The listing builds one solid part. Answer for the finished solid, in the listing's coordinates (mm). Face numbers are marked on the shaded views. A direction names the side the tool comes from. Give positions to 0.01 mm unless a question says otherwise; leave off trailing zeros. Write each loop counter-clockwise with the first axis right and the second up, starting at its lowest first coordinate (ties: lowest second). Pieces come first, ordered by that corner, then holes. Notation, with made-up numbers: (70, 85) -> (84, 85) arc R14 cw to (84, 111) -> close; hole circle Ø9 at (56, 27). An arc over 180 degrees is marked (long way). Put each result on its own line as item: value. Start each with the question number.
1) A cutting plane is placed at D-D (x = 5.25). Write down the section's boundary in (y, z) (3 decimals), then the cut area to 3 significant figures.
2) Find the intervals of material crossed by line 1 along Z through (x, y) = (0, -2); line 2 along Z through (x, y) = (0.5, -2.25); line 3 along Z through (x, y) = (5, 3.25), in increasing order. Write a range as from..to.
3) A cutting plane is placed at C-C (z = -3.5). Write down the section's boundary in (x, y).
4) Flat-ended cylindrical pins translate along their axes: pin 1 Ø6 at (x, z) = (0, -40.259) entering from -Y (3 decimals); pin 2 Ø1.5 at (x, y) = (2, -4) entering from -Z. Find the tip coordinate at first contact, or state that the pin passes through.
5) For a pull along Z with two mould halves and no side action, classify the marked faces 5, 6 and 7 as released by +Z, released by -Z, zero draft, split by the parting line, or undercut.
6) A cutting plane is placed at A-A (x = 0). Write down the section's boundary in (y, z) (3 decimals), then the cut area to 3 significant figures.
7) For the marked faces 1, 2, 3 and 4, determine the directions among +Z, -Z, +X, -X, +Y, -Y from which every point of the face is accessible in a straight line to the end or side of a thin tool.
8) A cutting plane is placed at B-B (y = 0). Write down the section's boundary in (x, z), then the cut area to 3 significant figures.
from build123d import *

# Parameters (mm, degrees)
SKETCH1_R           = 6.35
BOSS_EXTRUDE1_DEPTH = 11.049
SKETCH2_R           = 1.27
BOSS_EXTRUDE2_DEPTH = 22.86
FILLET1_R           = 1.27
SKETCH3_W           = 12.7
SKETCH3_H           = 6.35
BOSS_EXTRUDE3_DEPTH = 11.049
FILLET2_R           = 1.27
FILLET3_R           = 5.08
SKETCH4_R           = 2.3749
CUT_EXTRUDE1_DEPTH  = 10.525


with BuildPart() as part:
    # Sketch1 → Boss-Extrude1 (new body)
    with BuildSketch(Plane.XY):
        Circle(SKETCH1_R)
    extrude(amount=-BOSS_EXTRUDE1_DEPTH)

    # Sketch2 → Boss-Extrude2 (add)
    with BuildSketch(Plane(origin=(0, 0, -11.049), x_dir=(-1, 0, 0), z_dir=(0, 0, -1))):
        Circle(SKETCH2_R)
    extrude(amount=BOSS_EXTRUDE2_DEPTH)

    # Fillet1
    fillet1_edges = [part.edges().sort_by_distance(p)[0] for p in [
        (1.27, 0, -11.049),
    ]]
    fillet(fillet1_edges, radius=FILLET1_R)

    # Sketch3 → Boss-Extrude3 (add)
    with BuildSketch(Plane(origin=(0, 0, -33.909), x_dir=(-1, 0, 0), z_dir=(0, 0, -1))):
        Rectangle(SKETCH3_W, SKETCH3_H)
    extrude(amount=BOSS_EXTRUDE3_DEPTH)

    # Fillet2
    fillet2_edges = [part.edges().sort_by_distance(p)[0] for p in [
        (1.27, 0, -33.909),
    ]]
    fillet(fillet2_edges, radius=FILLET2_R)

    # Fillet3
    fillet3_edges = [part.edges().sort_by_distance(p)[0] for p in [
        (6.35, 0, -44.958),
        (-6.35, 0, -44.958),
    ]]
    fillet(fillet3_edges, radius=FILLET3_R)

    # Sketch4 → Cut-Extrude1 (cut, through all)
    with BuildSketch(Plane(origin=(0, 3.175, 0), x_dir=(1, 0, 0), z_dir=(0, 1, 0))):
        with Locations((0, 40.259)):
            Circle(SKETCH4_R)
    extrude(amount=-CUT_EXTRUDE1_DEPTH, mode=Mode.SUBTRACT)


solid = part.part
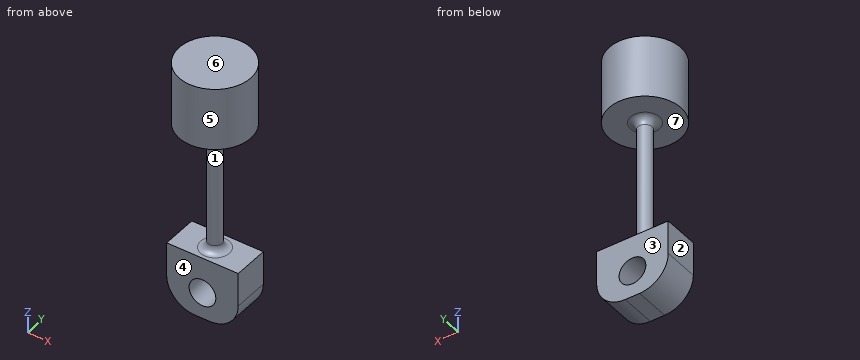
Reply:
1. outline: (-3.572, -11.049) -> (3.572, -11.049) -> (3.572, 0) -> (-3.572, 0) -> close; (-3.175, -43.035) -> (3.175, -43.035) -> (3.175, -33.909) -> (-3.175, -33.909) -> close
1. area: 137 mm2
2. line 1: z = -44.96..-42.63, -37.88..-33.79, -11.17..0
2. line 2: z = -44.96..-42.58, -37.94..-33.89, -11.07..0
2. line 3: z = -11.05..0
3. outline: circle Ø12.7 at (0, 0)
4. pin 1: stops at y = -3.175
4. pin 2: stops at z = -11.05
5. face 5: zero draft
5. face 6: released by +Z
5. face 7: undercut
6. outline: (-6.35, -11.049) -> (-2.54, -11.049) arc R1.27 cw to (-1.27, -12.319) -> (-1.27, -32.639) arc R1.27 cw to (-2.54, -33.909) -> (-3.175, -33.909) -> (-3.175, -37.884) -> (3.175, -37.884) -> (3.175, -33.909) -> (2.54, -33.909) arc R1.27 cw to (1.27, -32.639) -> (1.27, -12.319) arc R1.27 cw to (2.54, -11.049) -> (6.35, -11.049) -> (6.35, 0) -> (-6.35, 0) -> close; (-3.175, -44.958) -> (3.175, -44.958) -> (3.175, -42.634) -> (-3.175, -42.634) -> close
6. area: 240 mm2
7. face 1: none
7. face 2: +Z, -Z, -X, +Y, -Y
7. face 3: -Z, +X, -X, +Y
7. face 4: -Z, +X, -X, -Y
8. outline: (-6.35, -39.88) arc R5.08 ccw to (-1.27, -44.96) -> (1.27, -44.96) arc R5.08 ccw to (6.35, -39.88) -> (6.35, -33.91) -> (2.54, -33.91) arc R1.27 cw to (1.27, -32.64) -> (1.27, -12.32) arc R1.27 cw to (2.54, -11.05) -> (6.35, -11.05) -> (6.35, 0) -> (-6.35, 0) -> (-6.35, -11.05) -> (-2.54, -11.05) arc R1.27 cw to (-1.27, -12.32) -> (-1.27, -32.64) arc R1.27 cw to (-2.54, -33.91) -> (-6.35, -33.91) -> close; hole circle Ø4.75 at (0, -40.26)
8. area: 311 mm2
